```python
from build123d import *

# Parameters (mm, degrees)
BOSS_EXTRUDE1_DEPTH = 40
SKETCH2_R           = 1.65
BOSS_EXTRUDE2_DEPTH = 2
FILLET2_R           = 2


with BuildPart() as part:
    # Sketch1 → Boss-Extrude1 (new body)
    with BuildSketch(Plane(origin=(0, 0, 0), x_dir=(1, 0, 0), z_dir=(0, 1, 0))):
        Polygon((-2.5, -13.75), (2.5, -13.75), (2.5, -2.5), (13.75, -2.5), (13.75, 2.5), (2.5, 2.5), (2.5, 13.75), (-2.5, 13.75), (-2.5, 2.5), (-13.75, 2.5), (-13.75, -2.5), (-2.5, -2.5), align=None)
    extrude(amount=BOSS_EXTRUDE1_DEPTH)

    # Sketch2 → Boss-Extrude2 (add)
    with BuildSketch(Plane(origin=(0, 40, 0), x_dir=(1, 0, 0), z_dir=(0, 1, 0))):
        with Locations(Location((0, 0, 0), (0, 0, 270))):
            Circle(SKETCH2_R)
        with Locations(Location((11.25, 0, 0), (0, 0, 270))):
            Circle(SKETCH2_R)
        with Locations(Location((-11.25, 0, 0), (0, 0, 270))):
            Circle(SKETCH2_R)
        with Locations(Location((0, 11.25, 0), (0, 0, 270))):
            Circle(SKETCH2_R)
        with Locations(Location((0, -11.25, 0), (0, 0, 270))):
            Circle(SKETCH2_R)
    extrude(amount=BOSS_EXTRUDE2_DEPTH)

    # Fillet2
    fillet2_edges = [part.edges().sort_by_distance(p)[0] for p in [
        (13.75, 0, 0),
        (8.125, 0, 2.5),
        (2.5, 0, 8.125),
        (0, 0, 13.75),
        (-2.5, 0, 8.125),
        (-8.125, 0, 2.5),
        (-13.75, 0, 0),
        (-8.125, 0, -2.5),
        (-2.5, 0, -8.125),
        (0, 0, -13.75),
        (2.5, 0, -8.125),
        (8.125, 0, -2.5),
    ]]
    fillet(fillet2_edges, radius=FILLET2_R)


solid = part.part
```
The listing builds one solid part. Answer for the finished solid, in the listing's coordinates (mm). A direction names the side the tool comes from. Give positions to 0.01 mm unless a question says otherwise; leave off trailing zeros. Write each loop counter-clockwise with the first axis right and the second up, starting at its lowest first coordinate (ties: lowest second). Pieces come first, ordered by that corner, then holes. Notation, with made-up numbers: (-30, -15) -> (2, -15) arc R30 ccw to (2, 13) -> close; hole circle Ø5 at (71.5, -33.5). An arc over 180 degrees is marked (long way). Write item = value, one per line. Start each with the question number.
1) Straight lines are drawn through the part: line 1 along Z through (x, y) = (-6.5, 19); line 2 along Y through (x, z) = (3, -0.25). For each, find the intervals that lie inside material, in ascending order.
2) The part is cut by section A-A, the plane z = 0. Determine the outline of the cut face in (x, y), and give its area (3 significant figures).
3) Each of these flat-tipped pins is pushed along its axis until it touches: pin 1 (10 mm diameter, centred on x = -10.5, y = 13.5, fed in from -Z); pin 2 (5.5 mm diameter, centred on y = 20, z = -7.5, fed in from -X); pin 3 (10 mm diameter, centred on y = 20, z = -8, fed in from +X). Where does it stop, or does it pass through?
4) The part is cut by section B-B, the plane x = 0. Determine the outline of the cut face in (y, z), and give its area (3 significant figures).
5) Which of the six approach directions +Z, -Z, +X, -X, +Y, -Y give full straight-line access (tool end or side, diameter ignored) to faces 1 (the face through (-2.5, 21, -8)), 2 (the face through (-1.9, 0.57, -7.03)), 3 (the face through (-12.86, 40.99, -0.36)), 4 (the face through (8, 21, -2.5))?
6) The part is cut by section D-D, the plane x = 3. Determine the outline of the cut face in (y, z), and give its area (3 significant figures).
7) Determine the mould class of faces 5 (the face through (7.03, 0.57, -1.9)), 6 (the face through (0, 42, 0)), 7 (the face through (-2, 40, 1)) for opening direction Z: +Z half, -Z half, draft (parallel to the pull), parting line (faces both ways), or undercut.
8) The part is cut by section C-C, the plane y = 9. Determine the outline of the cut face in (x, z).
Solutions:
q1.line_1 = -2.5 to 2.5
q1.line_2 = 0 to 40
q2.outline = (-13.75, 2) arc R2 ccw to (-11.75, 0) -> (11.75, 0) arc R2 ccw to (13.75, 2) -> (13.75, 40) -> (12.9, 40) -> (12.9, 42) -> (9.6, 42) -> (9.6, 40) -> (1.65, 40) -> (1.65, 42) -> (-1.65, 42) -> (-1.65, 40) -> (-9.6, 40) -> (-9.6, 42) -> (-12.9, 42) -> (-12.9, 40) -> (-13.75, 40) -> close
q2.area = 1,120 mm²
q3.pin_1 = -2.5
q3.pin_2 = -2.5
q3.pin_3 = 2.5
q4.outline = (0, -11.75) arc R2 ccw to (2, -13.75) -> (40, -13.75) -> (40, -12.9) -> (42, -12.9) -> (42, -9.6) -> (40, -9.6) -> (40, -1.65) -> (42, -1.65) -> (42, 1.65) -> (40, 1.65) -> (40, 9.6) -> (42, 9.6) -> (42, 12.9) -> (40, 12.9) -> (40, 13.75) -> (2, 13.75) arc R2 ccw to (0, 11.75) -> close
q4.area = 1,120 mm²
q5.face_1 = -Z, -X, +Y, -Y
q5.face_2 = -Z, -X, -Y
q5.face_3 = +Y
q5.face_4 = -Z, +X, +Y, -Y
q6.outline = (0, -0.5) arc R2 ccw to (2, -2.5) -> (40, -2.5) -> (40, 2.5) -> (2, 2.5) arc R2 ccw to (0, 0.5) -> close
q6.area = 198 mm²
q7.face_5 = -Z half
q7.face_6 = draft
q7.face_7 = undercut
q8.outline = (-13.75, -2.5) -> (-2.5, -2.5) -> (-2.5, -13.75) -> (2.5, -13.75) -> (2.5, -2.5) -> (13.75, -2.5) -> (13.75, 2.5) -> (2.5, 2.5) -> (2.5, 13.75) -> (-2.5, 13.75) -> (-2.5, 2.5) -> (-13.75, 2.5) -> close
